Can you work these out from the drawing? Everything is in mm from the part's minimum corner. A direction names the side the tool comes from. Give positions to 0.01 mm unless a question says otherwise; leave off trailing zeros. Loops run counter-clockwise (first coordinate to the right, second up) from the corner with the lowest first, then second, coordinate; pieces in that order, holes last. Notation, with made-up numbers: (43, -19.75) - (95, -19.75) arc R28 cw to (95, 6.25) - close; hole circle Ø6 at (27, 36). An arc over 180 degrees is marked (long way). Answer in a Markdown table with one row per item.
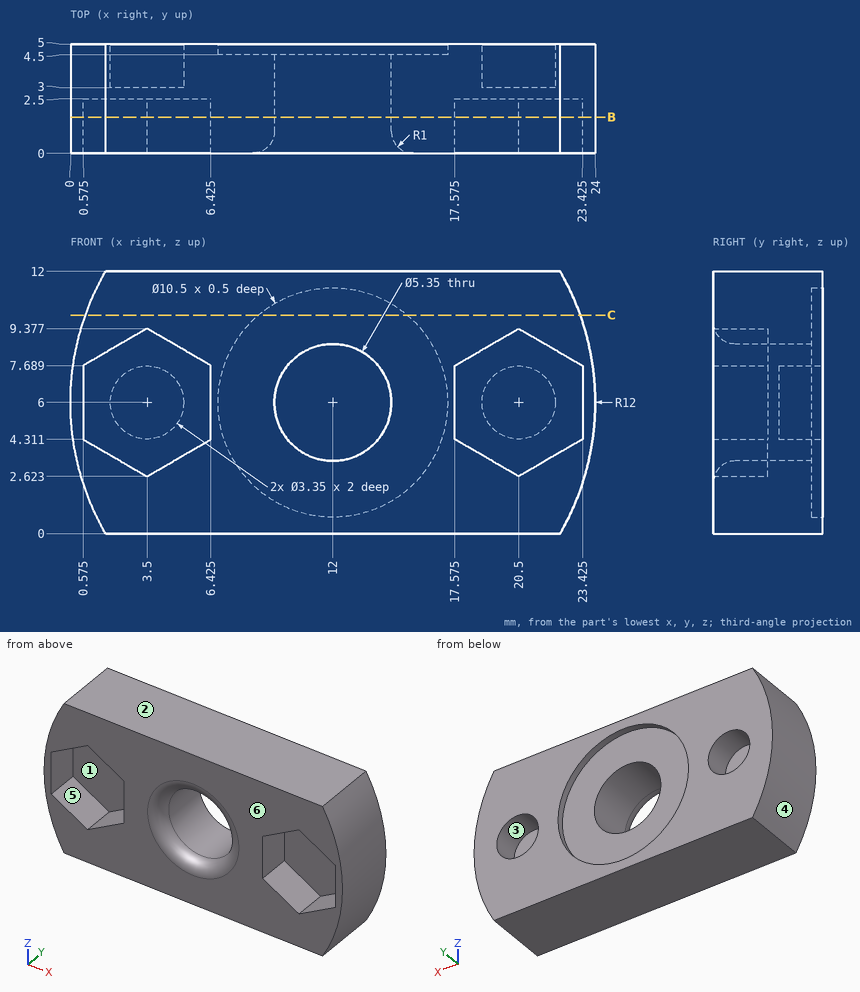
Q1. If we mould it in two halves opening along Z, with no side actions, what happens to the marked faces 4, 5 and 6? For each: released by +Z, released by -Z, zero draft, split by the parting line, or undercut.
Checked values:
| item | result |
|---|---|
| face 4 | split by the parting line |
| face 5 | undercut |
| face 6 | zero draft |
Q2. If I drill on line 1 (Z direction, x = 3.5, y = 4.5) (1 decimal); line 2 (Z direction, x = 12, y = 3.35) (1 decimal); line 3 (Y direction, x = 15.5, z = 2.5), over which ranges is the centre line in solid material (lowest first)? Write a range as [from, to].
Checked values:
| item | result |
|---|---|
| line 1 | z = [0, 4.3], [7.7, 12] |
| line 2 | z = [0, 3.3], [8.7, 12] |
| line 3 | y = [0, 4.5] |
Q3. Imagine slicing it at B-B, the plane y = 1.65. Count the separate pieces of the cut face and the enclosed holes in it, and give its area (3 significant figures).
Checked values:
| item | result |
|---|---|
| separate pieces | 1 |
| enclosed holes | 3 |
| area | 194 mm² |
Q4. On a 3-axis mill with a long thin cutter (end or side, diameter ignored), from which of +Z, -Z, +X, -X, +Y, -Y can I reach the whole of each face in a straight line? I mean the marked faces 1, 2 and 3. Say none if no direction works.
Checked values:
| item | result |
|---|---|
| face 1 | -Y |
| face 2 | +Z, +X, -X, +Y, -Y |
| face 3 | +Y |
Q5. For pin 1 (1.7 mm diameter, centred on x = 20, z = 5.5, fed in from +Y); pin 2 (3 mm diameter, centred on x = 20.5, z = 6, fed in from -Y); pin 3 (3 mm diameter, centred on y = 2, z = 2.5, fed in from -X), each with a flat end and sliding along its axis, tell me the tip position at first contact or that it passes through.
Checked values:
| item | result |
|---|---|
| pin 1 | stops at y = 3 |
| pin 2 | stops at y = 2.5 |
| pin 3 | stops at x = 0.17 |
Q6. Imagine slicing it at C-C, the plane z = 10. Write out the boundary of the cut face in (x, y), and give its area (3 significant figures).
Checked values:
| item | result |
|---|---|
| outline | (0.69, 0) - (23.31, 0) - (23.31, 5) - (15.4, 5) - (15.4, 4.5) - (8.6, 4.5) - (8.6, 5) - (0.69, 5) - close |
| area | 110 mm² |
